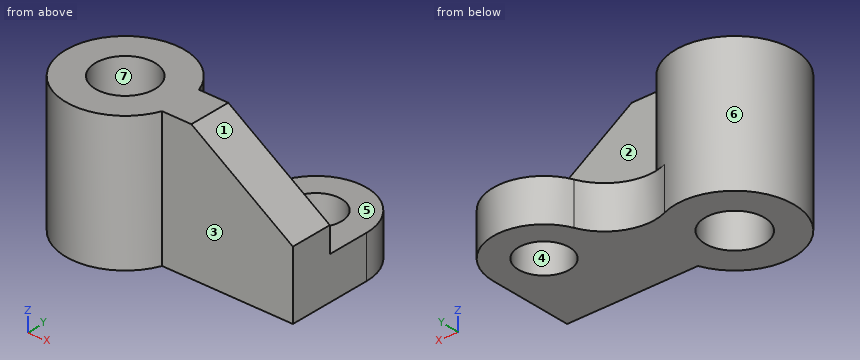
```python
from build123d import *

# Parameters (mm, degrees)
SKETCH1_R           = 7
BOSS_EXTRUDE1_DEPTH = 32
SKETCH1_3_R         = 6
BOSS_EXTRUDE2_DEPTH = 10
CHAMFER1_SIZE       = 16
CHAMFER1_SIZE2      = 24


with BuildPart() as part:
    # Sketch1 → Boss-Extrude1 (new body)
    with BuildSketch(Plane.XY):
        with BuildLine():
            Line((13.076696831, 5), (44, 5))
            Line((44, 5), (44, -5))
            Line((44, -5), (13.076696831, -5))
            ThreePointArc((13.076696831, -5), (-14, 0), (13.076696831, 5))
        make_face()
        Circle(SKETCH1_R, mode=Mode.SUBTRACT)
    extrude(amount=BOSS_EXTRUDE1_DEPTH)

    # Sketch1_3 → Boss-Extrude2 (add)
    with BuildSketch(Plane.XY):
        with BuildLine():
            ThreePointArc((20.893525638, 19.543811973), (14.440852002, 13.026785876), (5.269950687, 12.970259047))
            ThreePointArc((5.269950687, 12.970259047), (10.001556184, 9.796370445), (13.076696831, 5))
            Line((13.076696831, 5), (20, 5))
            Line((20, 5), (44, 5))
            Line((44, 5), (44, 15))
            ThreePointArc((44, 15), (34.315416556, 26.774499827), (20.893525638, 19.543811973))
        make_face()
        with Locations((32, 15)):
            Circle(SKETCH1_3_R, mode=Mode.SUBTRACT)
    extrude(amount=BOSS_EXTRUDE2_DEPTH)

    # Chamfer1
    chamfer1_edges = [part.edges().sort_by_distance(p)[0] for p in [
        (44, 0, 32),
    ]]
    chamfer1_side = [part.faces().sort_by_distance(p)[0] for p in [
        (44, 2.380952381, 13.380952381),
    ]]
    chamfer(chamfer1_edges, length=CHAMFER1_SIZE, length2=CHAMFER1_SIZE2, reference=chamfer1_side[0])


solid = part.part
```
Geometry check sheet. Reference: the model listing, model coordinates, mm. Face numbers are marked on the shaded views. A direction names the side the tool comes from. Coordinates: 2 decimals unless noted, no trailing zeros. Loops run counter-clockwise (first coordinate to the right, second up) from the corner with the lowest first, then second, coordinate; pieces in that order, holes last. Notation, with made-up numbers: (36, 7) -> (67, 7) arc R17 ccw to (67, 13) -> close; hole circle Ø3 at (57, -16). An arc over 180 degrees is marked (long way). Put each result on its own line as item: value.
1) Cross-section at B-B on z = 28. Record the boundary of the cut face in (x, y).
Result set:
outline: (13.08, -5) -> (26, -5) -> (26, 5) -> (13.08, 5) arc R14 ccw (long way) to start; hole circle Ø14 at (0, 0)
2) Cross-section at C-C on y = 0. Record the boundary of the cut face in (x, z), plus the area to 3 significant figures.
Result set:
outline: (-14, 0) -> (-7, 0) -> (-7, 32) -> (-14, 32) -> close; (7, 0) -> (44, 0) -> (44, 16) -> (20, 32) -> (7, 32) -> close
area: 1,220 mm^2
3) Gauge pin test, flat ends, axial feed: pin 1 Ø17.5 at (x, z) = (31, 16) entering from +Y; pin 2 Ø3 at (x, y) = (38, 11.5) entering from +Z; pin 3 Ø3 at (y, z) = (-10, 13.5) entering from +X; pin 4 Ø12.5 at (x, y) = (0, 0) entering from -Z. Record the tip position at first contact, or that the pin passes through.
Result set:
pin 1: stops at y = 27
pin 2: stops at z = 10
pin 3: stops at x = 11.12
pin 4: passes through
4) Cross-section at D-D on z = 6.5. Record the boundary of the cut face in (x, y), plus the area to 3 significant figures.
Result set:
outline: (5.27, 12.97) arc R14 ccw (long way) to (13.08, -5) -> (44, -5) -> (44, 15) arc R12 ccw to (20.89, 19.54) arc R12 cw to start; hole circle Ø14 at (0, 0); hole circle Ø12 at (32, 15)
area: 1,200 mm^2
5) Thickness scan on line 1 (Y direction, x = 0, z = 18); line 2 (Y direction, x = 32, z = 6); line 3 (Z direction, x = 39.5, y = 13). Record the ranges inside material, lowest first.
Result set:
line 1: y = -14 to -7, 7 to 14
line 2: y = -5 to 9, 21 to 27
line 3: z = 0 to 10
6) Cross-section at A-A on x = 32. Record the boundary of the cut face in (y, z), plus the area to 3 significant figures.
Result set:
outline: (-5, 0) -> (9, 0) -> (9, 10) -> (5, 10) -> (5, 24) -> (-5, 24) -> close; (21, 0) -> (27, 0) -> (27, 10) -> (21, 10) -> close
area: 340 mm^2
7) Release check for a two-part mould opening along Y. For the marked faces 4, 5, 6 and 7 record: released by +Y, released by -Y, zero draft, split by the parting line, or undercut.
Result set:
face 4: undercut
face 5: zero draft
face 6: split by the parting line
face 7: undercut
8) Tool access check on the marked faces 1, 2 and 3. Record the directions out of +Z, -Z, +X, -X, +Y, -Y that give a thin tool (end or side, any length) a straight path to the whole face; none if there is none.
Result set:
face 1: +Z, +X, +Y, -Y
face 2: +Z, +X, +Y
face 3: +Z, -Z, +X, -Y
